Answer from the drawing. Dimensions are ordinates in mm from the lowest x, y and z of the part. Coordinates: 2 decimals unless noted, no trailing zeros. Order: outer loops, then holes, each group sorted by start corner. A loop starts at its lowest first (then second) coordinate and runs counter-clockwise, first axis right, second up.
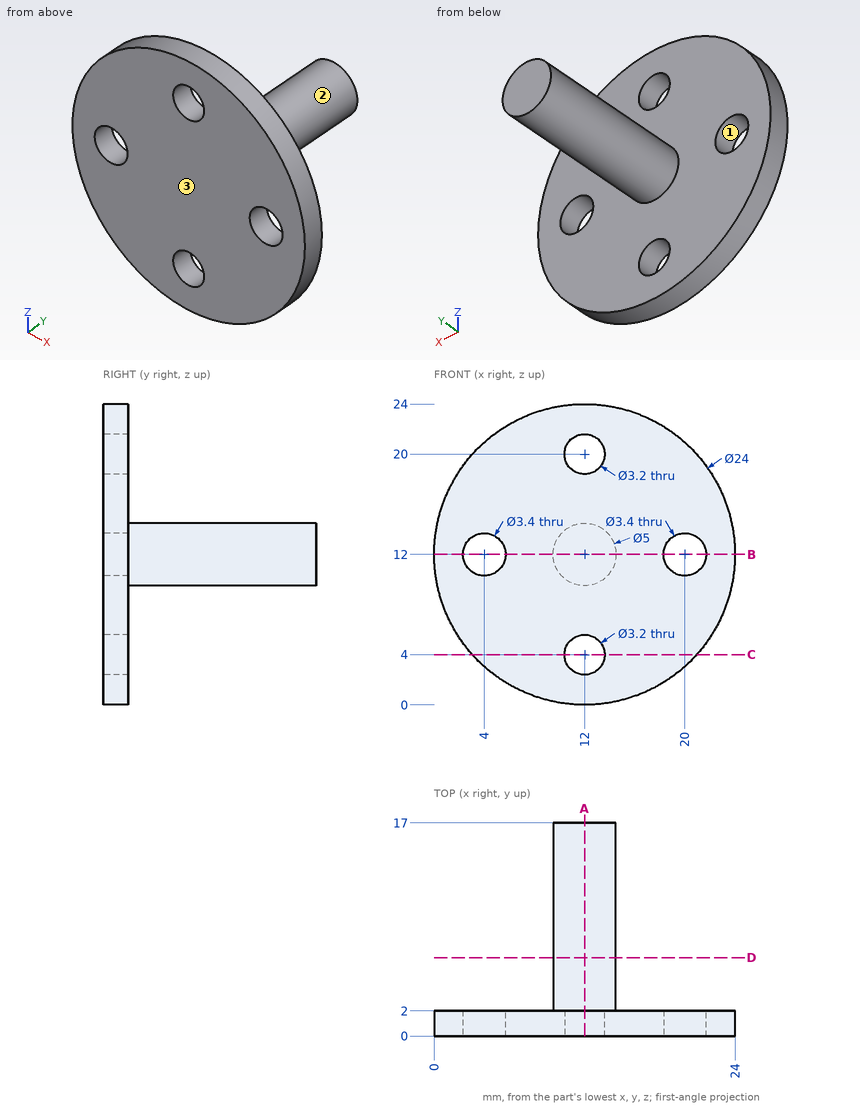
1) Section C-C (z = 4) is taken. Give the vertices of the cut face in (x, y).
2) Section B-B (z = 12) is taken. Give the vertices of the cut face in (x, y), then the cut area to 3 significant figures.
3) Determine the mould class of the marked faces 1, 2 and 3 for opening direction X: released by +X, released by -X, zero draft, split by the parting line, or undercut.
4) Consider L1, parallel to X at y = 1.6, z = 12; L2, parallel to Z at x = 12, y = 1.3; L3, parallel to Y at x = 10.25, z = 1.5. Determine where each line is inside the solid, lowest interval first.
5) Section D-D (y = 6.25) is taken. Give the vertices of the cut face in (x, z).
6) Section A-A (x = 12) is taken. Give the vertices of the cut face in (y, z).
7) Each of these flat-tipped pins is pushed along its axis until it touches: P1, Ø8, axis at x = 12.5, y = 6.5, coming from the -Z side; P2, Ø3.5, axis at x = 12, z = 20, coming from the +Y side; P3, Ø4, axis at x = 21, y = 4.5, coming from the +Z side. Where does it stop, or does it pass through?
Filled sheet:
1. outline: (3.06, 0) - (10.4, 0) - (10.4, 2) - (3.06, 2) - close; (13.6, 0) - (20.94, 0) - (20.94, 2) - (13.6, 2) - close
2. outline: (0, 0) - (2.3, 0) - (2.3, 2) - (0, 2) - close; (5.7, 0) - (18.3, 0) - (18.3, 2) - (14.5, 2) - (14.5, 17) - (9.5, 17) - (9.5, 2) - (5.7, 2) - close; (21.7, 0) - (24, 0) - (24, 2) - (21.7, 2) - close
2. area: 109 mm2
3. face 1: undercut
3. face 2: split by the parting line
3. face 3: zero draft
4. L1: x = 0 to 2.3, 5.7 to 18.3, 21.7 to 24
4. L2: z = 0 to 2.4, 5.6 to 18.4, 21.6 to 24
4. L3: y = 0 to 2
5. outline: circle Ø5 at (12, 12)
6. outline: (0, 0) - (2, 0) - (2, 2.4) - (0, 2.4) - close; (0, 5.6) - (2, 5.6) - (2, 9.5) - (17, 9.5) - (17, 14.5) - (2, 14.5) - (2, 18.4) - (0, 18.4) - close; (0, 21.6) - (2, 21.6) - (2, 24) - (0, 24) - close
7. P1: stops at z = 9.5
7. P2: stops at y = 2
7. P3: passes through
